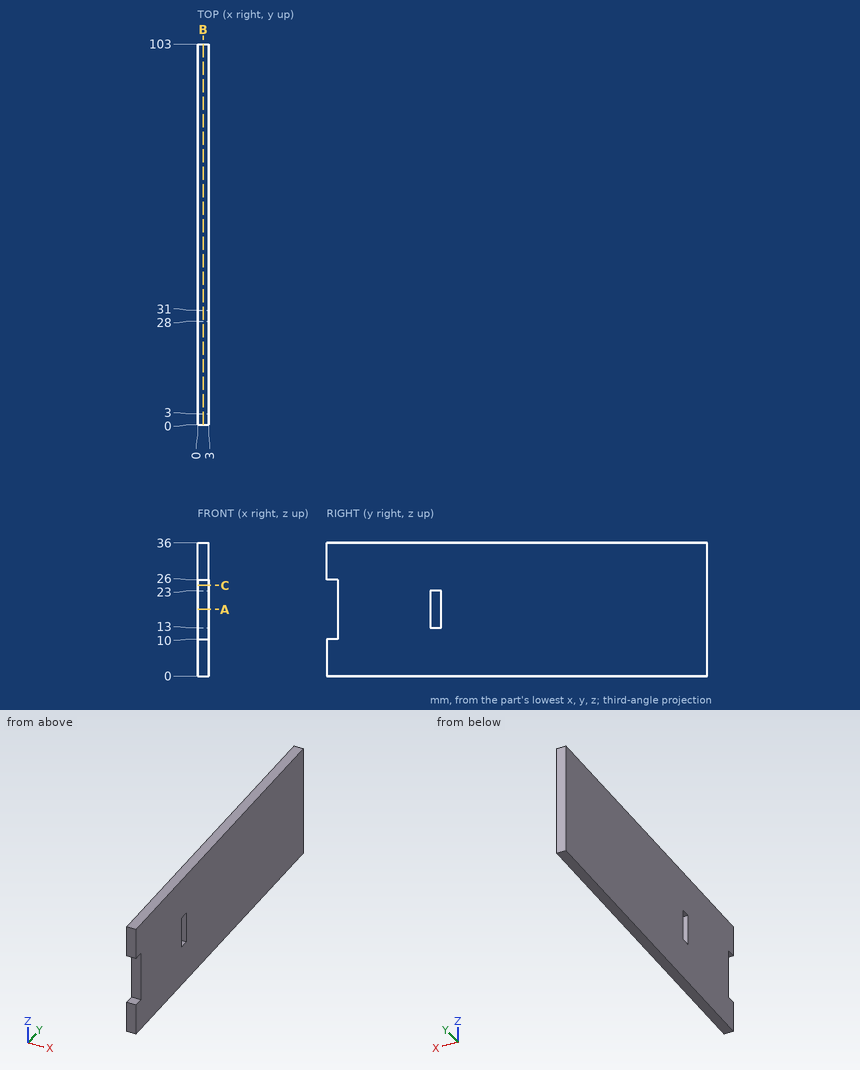
Geometry: see drawing. Coordinates: mm, zero at the bounding-box minimum. Coordinates: 2 decimals unless noted, no trailing zeros. Order: outer loops, then holes, each group sorted by start corner. A loop starts at its lowest first (then second) coordinate and runs counter-clockwise, first axis right, second up. Notation, with made-up numbers: M 3,-33.5 L 42,-33.5 A12 cw 42,-19.5 Z; hole C 53,38 d1. An arc over 180 degrees is marked long. Answer in a Markdown table with one row per item. Add a question column.
Q1. Line query: L1, parallel to Y at x = 1.1, z = 14; L2, parallel to Y at x = 1, z = 11.5. Output: solid intervals per line, ascending.
Q2. Section query B-B on x = 1.55. Return the cut outline in (y, z), and give its area (3 significant figures).
Q3. Section query C-C on z = 24.5. Return the cut outline in (x, y).
Q4. Section query A-A on z = 18. Return the cut outline in (x, y), and give its area (3 significant figures).
Completed:
| question | item | result |
|---|---|---|
| 1 | L1 | y = 3 to 28, 31 to 103 |
| 1 | L2 | y = 3 to 103 |
| 2 | outline | M 0,0 L 103,0 L 103,36 L 0,36 L 0,26 L 3,26 L 3,10 L 0,10 Z; hole M 28,13 L 31,13 L 31,23 L 28,23 Z |
| 2 | area | 3,630 mm2 |
| 3 | outline | M 0,3 L 3,3 L 3,103 L 0,103 Z |
| 4 | outline | M 0,3 L 3,3 L 3,28 L 0,28 Z; M 0,31 L 3,31 L 3,103 L 0,103 Z |
| 4 | area | 291 mm2 |
